from build123d import *

# Parameters (mm, degrees)
BOSS_EXTRU_1_DEPTH = 1.4
ESQUISSE2_R        = 1.25
BOSS_EXTRU_2_DEPTH = 1.1


with BuildPart() as part:
    # Esquisse1 → Boss.-Extru.1 (new body)
    with BuildSketch(Plane.XY):
        Polygon((-3.25, 0.75), (-3.25, 3.25), (-0.75, 3.25), (-0.75, 3.15), (0.75, 3.15), (0.75, 3.25), (3.25, 3.25), (3.25, 0.75), (3.15, 0.75), (3.15, -0.75), (3.25, -0.75), (3.25, -3.25), (0.75, -3.25), (0.75, -3.15), (-0.75, -3.15), (-0.75, -3.25), (-3.25, -3.25), (-3.25, -0.75), (-3.15, -0.75), (-3.15, 0.75), align=None)
    extrude(amount=BOSS_EXTRU_1_DEPTH)

    # Esquisse2 → Boss.-Extru.2 (add)
    with BuildSketch(Plane.XY.offset(1.4)):
        with Locations(Location((0, 0, 0), (0, 0, 180))):
            Circle(ESQUISSE2_R)
    extrude(amount=BOSS_EXTRU_2_DEPTH)


solid = part.part
Part model, mm, in its own coordinate system. A direction names the side the tool comes from. Coordinates: 2 decimals unless noted, no trailing zeros. Loops run counter-clockwise (first coordinate to the right, second up) from the corner with the lowest first, then second, coordinate; pieces in that order, holes last. Notation, with made-up numbers: (86, 31) - (112, 31) arc R12 cw to (112, 40) - close; hole circle Ø4 at (53, -26.75). An arc over 180 degrees is marked (long way). Write each question's results on one line, items separated by ' | '. Start each with the question number.
Q1. Probe line 1 along Y through (x, z) = (0, 2.3); line 2 along Y through (x, z) = (-1, 1.5); line 3 along Z through (x, y) = (0.5, 2.25). List the from-to ranges inside material, lowest first.
Q2. Drop flat-ended pins along their axis: pin 1 Ø2 at (x, y) = (1, -1.5) entering from +Z; pin 2 Ø0.7 at (y, z) = (0, 0.5) entering from -X; pin 3 Ø1.5 at (x, y) = (-0.5, 2.5) entering from +Z. Give the stop position or say it passes through.
Q3. Slice it at A-A on y = 0. Give the cut face in (x, z).
Q4. Slice it at D-D on y = 2. Give the cut face in (x, z).
Q5. Slice it at C-C on z = 1.85. Give the cut face in (x, y).
Q6. Two-plate mould, pull along X, no slides. Class faces 5 (the flat face through (0, -3.15, 1)), 6 (the cylindrical face through (1.25, -0.05, 1.94)), 7 (the flat face through (-3.25, 2, 1)): +X half, -X half, draft (parallel to the pull), parting line (faces both ways), or undercut.
Q7. Which spindle directions (+Z, -Z, +X, -X, +Y, -Y) get a long thin tool onto all of the face, cutting with end or side? Do faces 1 (the flat face through (3.15, 0, 1)), 2 (the flat face through (1.5, 0, 1.4)), 3 (the flat face through (-3.15, 0, 1)), 4 (the flat face through (0, 3.15, 1)). Say none if no direction does.
Answer:
1) line 1: y = -1.25 to 1.25 | line 2: y = -0.75 to 0.75 | line 3: z = 0 to 1.4
2) pin 1: stops at z = 2.5 | pin 2: stops at x = -3.15 | pin 3: stops at z = 1.4
3) outline: (-3.15, 0) - (3.15, 0) - (3.15, 1.4) - (1.25, 1.4) - (1.25, 2.5) - (-1.25, 2.5) - (-1.25, 1.4) - (-3.15, 1.4) - close
4) outline: (-3.25, 0) - (3.25, 0) - (3.25, 1.4) - (-3.25, 1.4) - close
5) outline: circle Ø2.5 at (0, 0)
6) face 5: undercut | face 6: parting line | face 7: -X half
7) face 1: +Z, -Z, +X | face 2: +Z | face 3: +Z, -Z, -X | face 4: +Z, -Z, +Y
